The listing builds one solid part. Answer for the finished solid, in the listing's coordinates (mm). Face numbers are marked on the shaded views. A direction names the side the tool comes from. Coordinates: 2 decimals unless noted, no trailing zeros. Write each loop counter-clockwise with the first axis right and the second up, starting at its lowest first coordinate (ties: lowest second). Pieces come first, ordered by that corner, then holes. Notation, with made-up numbers: M 85.5,83.25 L 112.5,83.25 A23 ccw 112.5,96.25 Z; hole C 21,13 d5. An arc over 180 degrees is marked long. Put each result on its own line as item: value. Start each with the question number.
Autodesk Inventor part; units mm, degrees
ref_plane "YZ Plane" through (0, 0, 0) normal (1, 0, 0) x (0, 1, 0)
ref_plane "XZ Plane" through (0, 0, 0) normal (0, 1, 0) x (-1, 0, 0)
ref_plane "XY Plane" through (0, 0, 0) normal (0, 0, 1) x (1, 0, 0)
ref_plane "Work Plane1" through (0, 0, 0) normal (0, 0, 1) x (1, 0, 0)
sketch "Sketch1" plane through (0, 0, 0) normal (0, 0, 1) x (1, 0, 0)
  circle A0 centre (-13.5, -18.5) radius 3.15
  circle A1 centre (-13.5, 18.5) radius 3.15
  line L0 (-25, -23) -> (25, -23) construction
  line L1 (25, -23) -> (25, 23)
  line L2 (25, 23) -> (-25, 23) construction
  line L3 (-25, 23) -> (-25, -23) construction
  circle A2 centre (-15, 12) radius 2.65
  circle A3 centre (-15, -12) radius 2.65
  circle A4 centre (12, 0) radius 4.15
  line L4 (-25, -11.95) -> (-20, -11.95) construction
  line L5 (-20, -11.95) -> (-20, -7.95) construction
  line L6 (-20, -7.95) -> (-25, -7.95) construction
  line L7 (-25, 7.95) -> (-25, -7.95) construction
  line L8 (-25, 7.95) -> (-20, 7.95) construction
  line L9 (-20, 7.95) -> (-20, 11.95) construction
  line L10 (-20, 11.95) -> (-25, 11.95) construction
  line L11 (-25, 19.95) -> (-25, 11.95) construction
  line L12 (-25, 19.95) -> (-4, 19.95) construction
  line L13 (-4, 11.95) -> (-4, 19.95) construction
  line L14 (-4, 11.95) -> (-9, 11.95) construction
  line L15 (-9, 11.95) -> (-9, 7.95) construction
  line L16 (-9, 7.95) -> (-4, 7.95) construction
  line L17 (-4, -7.95) -> (-4, 7.95) construction
  line L18 (-4, -7.95) -> (-9, -7.95) construction
  line L19 (-9, -7.95) -> (-9, -11.95) construction
  line L20 (-9, -11.95) -> (-4, -11.95) construction
  line L21 (-4, -19.95) -> (-4, -11.95) construction
  line L22 (-4, -19.95) -> (-25, -19.95) construction
  line L23 (-25, -11.95) -> (-25, -19.95) construction
  line L24 (-4, -23.1) -> (-25, -23.1)
  line L25 (-25, -23.1) -> (-25, 23.1)
  line L26 (-25, 23.1) -> (-4, 23.1)
  line L27 (-4, 23.1) -> (-4, -23.1)
  point P0 (0, 0)
  dimension "d3" = 0.1
  dimension "d4" = 0.1
extrude "Extrusion1" add sketch "Sketch1" along normal blind 3 contours L24 L25 L26 L27
sketch "Sketch3" plane through (-25, 23.1, 0) normal (0, 1, 0) x (1, 0, 0)
  line L0 (50, 8.1) -> (0, 8.1) construction
  line L1 (0, 8.1) -> (0, 0.1) construction
  line L2 (50, 0.1) -> (0, 0.1) construction
  line L3 (50, 8.1) -> (50, 0.1) construction
  line L4 (21, 0) -> (0, 0) construction
  line L5 (0, 0) -> (0, -3) construction
  line L6 (21, -3) -> (0, -3) construction
  line L7 (21, 0) -> (21, -3) construction
  line L8 (21, -3) -> (0, -3)
  line L9 (0, -3) -> (50, -3)
  line L10 (50, -3) -> (50, 8.1)
  line L11 (50, 8.1) -> (0, 8.1)
  line L12 (0, 8.1) -> (0, -3)
  point P0 (25, 0)
extrude "Extrusion2" add sketch "Sketch3" along normal blind 100
sketch "Sketch5" plane through (-25, -23.1, 0) normal (-1, 0, 0) x (0, 0, 1)
  circle A0 centre (-2.55, 126.2) radius 2.65 construction
  circle A1 centre (-2.55, 106.2) radius 2.65 construction
  circle A2 centre (-2.55, 86.2) radius 2.65 construction
  circle A3 centre (-2.55, 66.2) radius 2.65 construction
  circle A4 centre (-2.55, 126.2) radius 2.5
  line L0 (-2.55, 126.2) -> (-2.55, 106.2) construction
  circle A5 centre (-2.55, 106.2) radius 2.5
  circle A6 centre (-2.55, 86.2) radius 2.5
  circle A7 centre (-2.55, 66.2) radius 2.5
  point P0 (0, 23.1)
  dimension "d17" = 5
  dimension "d20" = 20
extrude "Extrusion4" cut sketch "Sketch5" against normal blind 25
sketch "Sketch6" plane through (0, 0, 3) normal (0, 0, 1) x (1, 0, 0)
  circle A0 centre (4, 83.1) radius 2.65 construction
  circle A1 centre (4, 98.1) radius 2.65 construction
  circle A2 centre (4, 113.1) radius 2.65 construction
  circle A3 centre (4, 83.1) radius 2.5
  circle A4 centre (4, 98.1) radius 2.5
  circle A5 centre (4, 113.1) radius 2.5
  point P0 (0, 0)
  dimension "d27" = 5
  dimension "d28" = 5
  dimension "d29" = 5
extrude "Extrusion5" cut sketch "Sketch6" against normal through all
equation "\"d4\" = d3"
properties part number "endcap insert"
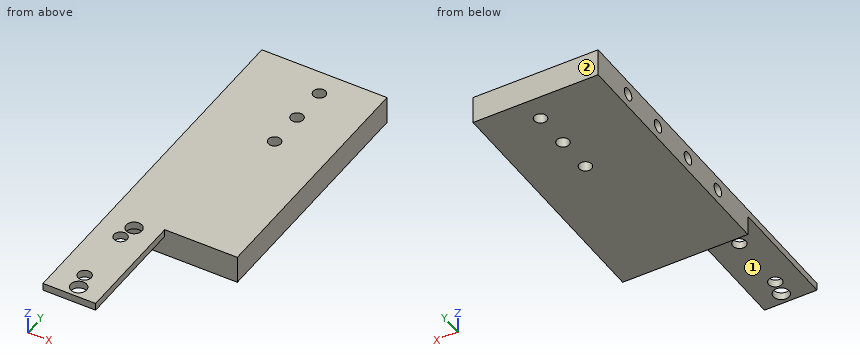
1) A cutting plane is placed at B-B on x = -14. State how many separate pieces and enclosed holes the cut face has, then the cut area to 3 significant figures.
2) For the marked faces 1 and 2, determine the directions among +Z, -Z, +X, -X, +Y, -Y from which every point of the face is accessible in a straight line to the end or side of a thin tool.
3) Given pin 1 Ø3 at (x, y) = (4, 83.1) entering from -Z; pin 2 Ø4 at (y, z) = (43, -3) entering from -X; pin 3 Ø7 at (x, y) = (-15, -12) entering from -Z; pin 4 Ø5.5 at (x, z) = (-6, -4) entering from -Y, each flat-ended and moving along its own axis, determine where each tip first touches the part or whether it passes through.
4) Straight lines are drawn through the part: probe 1 along Y at (x, z) = (-10, -2.55); probe 2 along Y at (x, z) = (5.5, -2.5); probe 3 along Y at (x, z) = (-13.5, 0.6). For each, find the intervals that lie inside material, in ascending order.
5) A cutting plane is placed at C-C on z = -3.25. Write down the section's boundary in (x, y).
6) A cutting plane is placed at D-D on y = 18.5. Write down the section's boundary in (x, z), then the cut area to 3 significant figures.
7) A cutting plane is placed at A-A on y = 83.1. Write down the section's boundary in (x, z), then the cut area to 4 significant figures.
Answers follow:
1. separate pieces: 5
1. enclosed holes: 4
1. area: 1,100 mm²
2. face 1: -Z, +X, -X, -Y
2. face 2: +Z, -Z, +X, -X, +Y
3. pin 1: passes through
3. pin 2: stops at x = 0
3. pin 3: stops at z = 0
3. pin 4: stops at y = 23.1
4. probe 1: y = 23.1 to 40.6, 45.6 to 60.6, 65.6 to 80.6, 85.6 to 100.6, 105.6 to 123.1
4. probe 2: y = 23.1 to 81.1, 85.1 to 96.1, 100.1 to 111.1, 115.1 to 123.1
4. probe 3: y = -23.1 to -21.65, -15.35 to -14.18, -9.82 to 9.82, 14.18 to 15.35, 21.65 to 123.1
5. outline: M -25,23.1 L 25,23.1 L 25,123.1 L -25,123.1 L -25,105.5 L 0,105.5 L 0,100.7 L -25,100.7 L -25,85.5 L 0,85.5 L 0,80.7 L -25,80.7 L -25,65.5 L 0,65.5 L 0,60.7 L -25,60.7 L -25,45.5 L 0,45.5 L 0,40.7 L -25,40.7 Z; hole C 4,83.1 d5; hole C 4,98.1 d5; hole C 4,113.1 d5
6. outline: M -25,0 L -16.65,0 L -16.65,3 L -25,3 Z; M -10.35,0 L -4,0 L -4,3 L -10.35,3 Z
6. area: 44.1 mm²
7. outline: M -25,-8.1 L 1.5,-8.1 L 1.5,3 L -25,3 L -25,-0.05 L 0,-0.05 L 0,-5.05 L -25,-5.05 Z; M 6.5,-8.1 L 25,-8.1 L 25,3 L 6.5,3 Z
7. area: 374.5 mm²
